```python
from build123d import *

# Parameters (mm, degrees)
BOSS_EXTRUDE1_DEPTH     = 10
CUT_EXTRUDE1_DEPTH      = 1
CUT_EXTRUDE1_DEPTH_BACK = 11
CUT_EXTRUDE2_DEPTH      = 11
LPATTERN1_COUNT         = 2
LPATTERN1_PITCH         = 31
LPATTERN1_COUNT_DIR2    = 2
LPATTERN1_PITCH_DIR2    = 31
SKETCH5_R               = 2.065
CUT_EXTRUDE3_DEPTH      = 11
SKETCH6_R               = 1.23
CUT_EXTRUDE4_DEPTH      = 8


with BuildPart() as part:
    # Sketch1 → Boss-Extrude1 (new body)
    with BuildSketch(Plane.XY):
        Polygon((348.8, 65), (350, 63.8), (350, 1.2), (348.8, 0), (1.2, 0), (0, 1.2), (0, 63.8), (1.2, 65), align=None)
    extrude(amount=BOSS_EXTRUDE1_DEPTH)

    # Sketch2 → Cut-Extrude1 (cut, two sides)
    with BuildSketch(Plane.XY.offset(10)) as cut_extrude1_sk:
        with BuildLine():
            Line((316, 33.5), (316, 0))
            Line((316, 0), (340, 0))
            Line((340, 0), (340, 33.5))
            ThreePointArc((340, 33.5), (328, 45.5), (316, 33.5))
        make_face()
    extrude(amount=CUT_EXTRUDE1_DEPTH, mode=Mode.SUBTRACT)
    extrude(cut_extrude1_sk.sketch, amount=-CUT_EXTRUDE1_DEPTH_BACK, mode=Mode.SUBTRACT)

    # Sketch3 → Cut-Extrude2 (cut, through all)
    with BuildSketch(Plane.XY.offset(10)):
        with BuildLine():
            Line((345.25, 16.5), (345.25, 8.5))
            ThreePointArc((345.25, 8.5), (343.5, 6.75), (341.75, 8.5))
            Line((341.75, 8.5), (341.75, 16.5))
            ThreePointArc((341.75, 16.5), (343.5, 18.25), (345.25, 16.5))
        make_face()
    cut_extrude2 = extrude(amount=-CUT_EXTRUDE2_DEPTH, mode=Mode.SUBTRACT)

    # LPattern1: Cut-Extrude2 2 × 2
    with Locations(*[(-j * LPATTERN1_PITCH_DIR2, i * LPATTERN1_PITCH, 0) for i in range(LPATTERN1_COUNT) for j in range(LPATTERN1_COUNT_DIR2) if (i, j) != (0, 0)]):
        add(cut_extrude2, mode=Mode.SUBTRACT)

    # Sketch5 → Cut-Extrude3 (cut, through all)
    with BuildSketch(Plane.XY.offset(10)):
        with Locations((328, 60)):
            Circle(SKETCH5_R)
        with Locations((12, 60)):
            Circle(SKETCH5_R)
        with Locations((297, 37)):
            Circle(SKETCH5_R)
        with BuildLine():
            Line((302, 61.25), (312, 61.25))
            ThreePointArc((312, 61.25), (314.25, 59), (312, 56.75))
            Line((312, 56.75), (302, 56.75))
            ThreePointArc((302, 56.75), (299.75, 59), (302, 61.25))
        make_face()
        with BuildLine():
            Line((242, 61.25), (252, 61.25))
            ThreePointArc((252, 61.25), (254.25, 59), (252, 56.75))
            Line((252, 56.75), (242, 56.75))
            ThreePointArc((242, 56.75), (239.75, 59), (242, 61.25))
        make_face()
    extrude(amount=-CUT_EXTRUDE3_DEPTH, mode=Mode.SUBTRACT)

    # Sketch6 → Cut-Extrude4 (cut)
    with BuildSketch(Plane(origin=(0, 65, 0), x_dir=(1, 0, 0), z_dir=(0, 1, 0))):
        with Locations((289.8, -5)):
            Circle(SKETCH6_R)
        with Locations((169.8, -5)):
            Circle(SKETCH6_R)
        with Locations((34.8, -5)):
            Circle(SKETCH6_R)
    extrude(amount=-CUT_EXTRUDE4_DEPTH, mode=Mode.SUBTRACT)


solid = part.part
```
The model under review builds one solid part; all positions refer to its coordinate system, in mm. A direction names the side the tool comes from. Give positions to 0.01 mm unless a question says otherwise; leave off trailing zeros. Loops run counter-clockwise (first coordinate to the right, second up) from the corner with the lowest first, then second, coordinate; pieces in that order, holes last. Notation, with made-up numbers: (-40, -22.75) - (-24, -22.75) arc R19 cw to (-24, -1.75) - close; hole circle Ø2 at (-19.5, -35). An arc over 180 degrees is marked (long way). Answer as a JSON object with one key per item and string values.
Q1. Insertion check: pin 1 (1.2 mm diameter, centred on x = 290, z = 5.5, fed in from +Y); pin 2 (4 mm diameter, centred on y = 14, z = 7.5, fed in from -X); pin 3 (3.5 mm diameter, centred on x = 328, y = 60, fed in from -Z). Each pin has a flat end and moves straight along its axis. Give the tip position at first contact, or say it passes through.
Worked out:
{"pin 1": "stops at y = 57", "pin 2": "stops at x = 0", "pin 3": "passes through"}
Q2. Add section A-A on y = 25. State the section outline as (x, z) points.
Worked out:
{"outline": "(0, 0) - (316, 0) - (316, 10) - (0, 10) - close; (340, 0) - (350, 0) - (350, 10) - (340, 10) - close"}
Q3. Mouldability with a two-part tool opening along X and no side actions: class faces 4 (the flat face through (0, 32, 5)), 5 (the flat face through (344, 0, 5)), 6 (the flat face through (307, 56.75, 5)), 7 (the flat face through (345.25, 13, 5)) as +X half, -X half, draft (parallel to the pull), parting line (faces both ways), or undercut.
Worked out:
{"face 4": "-X half", "face 5": "draft", "face 6": "undercut", "face 7": "undercut"}
Q4. To check wall thickness, follow line 1 along X through (y, z) = (59.5, 2.25); line 2 along Z through (x, y) = (169.8, 61.5); line 3 along Y through (x, z) = (296.5, 4). State the ranges of each line that lie inside material, in increasing order.
Worked out:
{"line 1": "x = 0 to 10, 14 to 239.81, 254.19 to 299.81, 314.19 to 326, 330 to 350", "line 2": "z = 0 to 3.77, 6.23 to 10", "line 3": "y = 0 to 35, 39 to 65"}
Q5. For faces 1 (the flat face through (341.75, 43, 5)), 2 (the flat face through (340, 17, 5)), 3 (the flat face through (350, 33, 5)), list the 3-axis set-ups (+Z, -Z, +X, -X, +Y, -Y) from which the entire face can be reached by the end or side of a thin tool; tool diameter is ignored.
Worked out:
{"face 1": "+Z, -Z", "face 2": "+Z, -Z, -Y", "face 3": "+Z, -Z, +X, +Y, -Y"}
